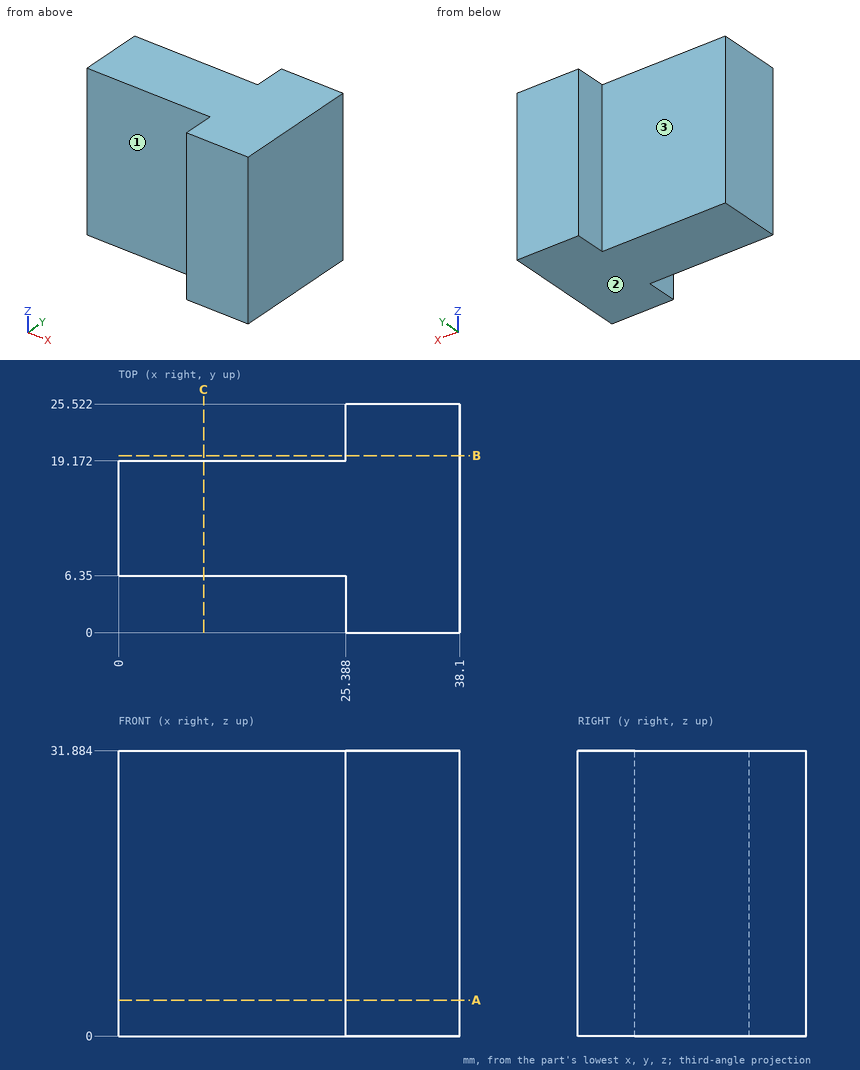
Here's the drawing with two shaded views (mm, measured from the low corner). I have some questions. A direction names the side the tool comes from. Round coordinates to 2 decimals unless told otherwise and drop trailing zeros. Order: outer loops, then holes, each group sorted by start corner. A loop starts at its lowest first (then second) coordinate and runs counter-clockwise, first axis right, second up. Notation, with made-up numbers: (18, -10.5) -> (37, -10.5) arc R29 cw to (37, 10.5) -> close; hole circle Ø11 at (-34, 67). An arc over 180 degrees is marked (long way). Return JSON: item names as keys, results as strings.
Q1. I need wall thicknesses on line 1 along Y through (x, z) = (20, 3); line 2 along X through (y, z) = (1, 14.5). Which ranges of each line are inside material? Lowest first, please. Write a range as from..to.
Filled sheet:
{"line 1": "y = 6.35..19.17", "line 2": "x = 25.39..38.1"}
Q2. Which directions (+Z, -Z, +X, -X, +Y, -Y) give clear straight access to the entire face, cutting with the end or side of a thin tool? Please do the marked faces 1, 2 and 3.
Filled sheet:
{"face 1": "+Z, -Z, -X, -Y", "face 2": "-Z, +X, -X, +Y, -Y", "face 3": "+Z, -Z, -X, +Y"}
Q3. For pin 1 Ø8 at (x, z) = (19.5, 7) entering from +Y; pin 2 Ø3 at (y, z) = (22, 14.5) entering from -X; pin 3 Ø7.5 at (x, z) = (10.5, 18.5) entering from -Y, each with a flat end and sliding along its axis, tell me the tip position at first contact or that it passes through.
Filled sheet:
{"pin 1": "stops at y = 19.17", "pin 2": "stops at x = 25.39", "pin 3": "stops at y = 6.35"}
Q4. If we section it at A-A on z = 4: List the corners of the cut face in (x, y) for me.
Filled sheet:
{"outline": "(0, 6.35) -> (25.39, 6.35) -> (25.39, 0) -> (38.1, 0) -> (38.1, 25.52) -> (25.39, 25.52) -> (25.39, 19.17) -> (0, 19.17) -> close"}
Q5. If we section it at B-B on y = 19.75: List the corners of the cut face in (x, z) for me.
Filled sheet:
{"outline": "(25.39, 0) -> (38.1, 0) -> (38.1, 31.88) -> (25.39, 31.88) -> close"}
Q6. If we section it at C-C on x = 9.5: List the corners of the cut face in (y, z) for me.
Filled sheet:
{"outline": "(6.35, 0) -> (19.17, 0) -> (19.17, 31.88) -> (6.35, 31.88) -> close"}
